The listing builds one solid part. Answer for the finished solid, in the listing's coordinates (mm). Give positions to 0.01 mm unless a question says otherwise; leave off trailing zeros. Write each loop counter-clockwise with the first axis right and the second up, starting at its lowest first coordinate (ties: lowest second). Pieces come first, ordered by that corner, then holes. Notation, with made-up numbers: (-19, -21.75) -> (-14, -21.75) arc R25 ccw to (-14, -6.75) -> close; hole circle Ø2 at (55.25, -34). An arc over 180 degrees is marked (long way). Put each result on its own line as item: value. Start each with the question number.
1) Flat-ended cylindrical pins translate along their axes: pin 1 Ø8 at (y, z) = (24, 150) entering from +X; pin 2 Ø12 at (x, z) = (29, 312.5) entering from +Y. Find the tip coordinate at first contact, or state that the pin passes through.
2) A cutting plane is placed at A-A (z = 306). Write down the section's boundary in (x, y).
3) Find the intervals of material crossed by line 1 along Y through (x, z) = (3.1, 270); line 2 along Y through (x, z) = (6.5, 207), in increasing order. Write a range as from..to.
4) A cutting plane is placed at B-B (x = 11). Write down the section's boundary in (y, z), then the cut area to 3 significant figures.
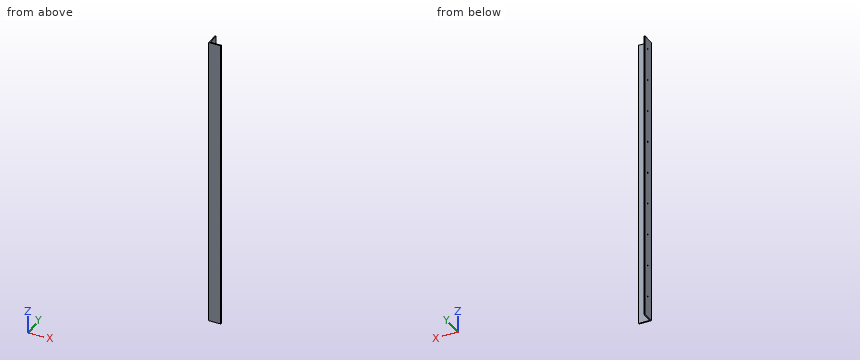
from build123d import *

# Parameters (mm, degrees)
BOSS_EXTRUDE1_DEPTH = 1080
SKETCH2_R           = 2.5
CUT_EXTRUDE1_DEPTH  = 1032.715076947


with BuildPart() as part:
    # Sketch1 → Boss-Extrude1 (new body)
    with BuildSketch(Plane(origin=(0, 0, -50), x_dir=(-1, 0, 0), z_dir=(0, 0, -1))):
        Polygon((0, 44), (-4, 44), (-4, 4), (-44, 4), (-44, 0), (0, 0), align=None)
    extrude(amount=-BOSS_EXTRUDE1_DEPTH)

    # Sketch2 → Cut-Extrude1 (cut, through all)
    with BuildSketch(Plane(origin=(4, 0, 0), x_dir=(0, 0, -1), z_dir=(1, 0, 0))):
        with Locations((-990, 24)):
            Circle(SKETCH2_R)
        with Locations((-870, 24)):
            Circle(SKETCH2_R)
        with Locations((-750, 24)):
            Circle(SKETCH2_R)
        with Locations((-630, 24)):
            Circle(SKETCH2_R)
        with Locations((-510, 24)):
            Circle(SKETCH2_R)
        with Locations((-390, 24)):
            Circle(SKETCH2_R)
        with Locations((-270, 24)):
            Circle(SKETCH2_R)
        with Locations((-150, 24)):
            Circle(SKETCH2_R)
        with Locations((-30, 24)):
            Circle(SKETCH2_R)
    extrude(amount=-CUT_EXTRUDE1_DEPTH, mode=Mode.SUBTRACT)


solid = part.part
Reply:
1. pin 1: stops at x = 4
1. pin 2: stops at y = 4
2. outline: (0, 0) -> (44, 0) -> (44, 4) -> (4, 4) -> (4, 44) -> (0, 44) -> close
3. line 1: y = 0..21.5, 26.5..44
3. line 2: y = 0..4
4. outline: (0, -50) -> (4, -50) -> (4, 1030) -> (0, 1030) -> close
4. area: 4,320 mm2
